Input: part model. Units: mm. Frame: model coordinates. A direction names the side the tool comes from. Give positions to 0.01 mm unless a question says otherwise; leave off trailing zeros. Order: outer loops, then holes, each group sorted by start corner. A loop starts at its lowest first (then second) coordinate and runs counter-clockwise, first axis right, second up. Notation, with made-up numbers: (18.5, 23) - (54.5, 23) arc R12 cw to (54.5, 41) - close; hole circle Ø7 at (-8, 12). An arc over 180 degrees is marked (long way). Use a Markdown table: item, result.
from build123d import *

# Parameters (mm, degrees)
PAD_DEPTH    = 6
SKETCH001_W  = 25
SKETCH001_H  = 3
PAD001_DEPTH = 15
FILLET_R     = 6
FILLET001_R  = 2


with BuildPart() as part:
    # Sketch → Pad (new body)
    with BuildSketch(Plane.XY):
        with BuildLine():
            Line((-12.5, 0), (12.5, 0))
            Line((12.5, 0), (12.5, 16))
            ThreePointArc((12.5, 16), (1.531208, 27.4461), (-11.884864, 19))
            Line((-11.884864, 19), (-3, 19))
            ThreePointArc((-4.898979, 16), (4.224745, 12.325765), (-3, 19))
            Line((-4.898979, 16), (-12.5, 16))
            Line((-12.5, 16), (-12.5, 0))
        make_face()
    extrude(amount=PAD_DEPTH)

    # Sketch001 → Pad001 (new body)
    with BuildSketch(Plane.XY.offset(6)):
        with Locations((0, 1.5)):
            Rectangle(SKETCH001_W, SKETCH001_H)
    extrude(amount=PAD001_DEPTH)

    # Fillet
    fillet_edges = [part.edges().sort_by_distance(p)[0] for p in [
        (0, 3, 6),
    ]]
    fillet(fillet_edges, radius=FILLET_R)

    # Fillet001
    fillet001_edges = [part.edges().sort_by_distance(p)[0] for p in [
        (-12.5, 1.5, 21),
        (12.5, 1.5, 21),
    ]]
    fillet(fillet001_edges, radius=FILLET001_R)


solid = part.part
1. Section query D-D (x = -7.75). Return loops of the section in (y, z), then the cut area to 3 significant figures.
Response:
| item | result |
|---|---|
| outline | (0, 0) - (16, 0) - (16, 6) - (9, 6) arc R6 cw to (3, 12) - (3, 21) - (0, 21) - close; (19, 0) - (24.86, 0) - (24.86, 6) - (19, 6) - close |
| area | 184 mm^2 |
2. Section query A-A (x = 0). Return loops of the section in (y, z), then the cut area to 3 significant figures.
Response:
| item | result |
|---|---|
| outline | (0, 0) - (10, 0) - (10, 6) - (9, 6) arc R6 cw to (3, 12) - (3, 21) - (0, 21) - close; (20, 0) - (27.54, 0) - (27.54, 6) - (20, 6) - close |
| area | 158 mm^2 |
3. Set-up query: faces 1 (the face through (-9, 16, 3)), 2 (the face through (1.769, 27.414, 2.958)), 3 (the face through (0, 3, 16)). Return all of +Z, -Z, +X, -X, +Y, -Y with unobstructed straight access to the full face (end or side cutting, diameter ignored); none if empty.
Response:
| item | result |
|---|---|
| face 1 | +Z, -Z, -X |
| face 2 | +Z, -Z, +Y |
| face 3 | +Z, +X, -X, +Y |
4. Pin query (flat end, axial travel): pin 1 (1.5 mm diameter, centred on x = -5.5, z = 13.5, fed in from +Y); pin 2 (4 mm diameter, centred on x = -3, y = 6, fed in from +Z); pin 3 (10 mm diameter, centred on x = -0.5, z = 15, fed in from +Y). Return the tip coordinate at first contact, or that it passes through.
Response:
| item | result |
|---|---|
| pin 1 | stops at y = 3 |
| pin 2 | stops at z = 8.68 |
| pin 3 | stops at y = 3.34 |
5. Section query C-C (z = 5). Return loops of the section in (x, y), then the cut area to 3 significant figures.
Response:
| item | result |
|---|---|
| outline | (-12.5, 0) - (12.5, 0) - (12.5, 16) arc R12.54 ccw to (-11.88, 19) - (-3, 19) arc R5 cw (long way) to (-4.9, 16) - (-12.5, 16) - close |
| area | 519 mm^2 |
6. Section query B-B (y = 15). Return loops of the section in (x, z), then the cut area to 3 significant figures.
Response:
| item | result |
|---|---|
| outline | (-12.5, 0) - (-5, 0) - (-5, 6) - (-12.5, 6) - close; (5, 0) - (12.5, 0) - (12.5, 6) - (5, 6) - close |
| area | 90.0 mm^2 |
7. Material intervals for line 1 along X through (y, z) = (15, 3.25); line 2 along Y through (x, z) = (0, 3.8); line 3 along Z through (x, y) = (7.25, 11), sorted ascending.
Response:
| item | result |
|---|---|
| line 1 | x = -12.5 to -5, 5 to 12.5 |
| line 2 | y = 0 to 10, 20 to 27.54 |
| line 3 | z = 0 to 6 |
